from build123d import *

# Parameters (mm, degrees)
SKETCH1_R                                            = 165
SKETCH1_R_2                                          = 132
BOSS_EXTRUDE1_DEPTH                                  = 15
M8_CLEARANCE_HOLE1_D                                 = 9
CIRPATTERN1_COUNT                                    = 6
SKETCH4_R                                            = 10
CUT_EXTRUDE1_DEPTH                                   = 4
CSK_FOR_M10_HEX_SOCKET_COUNTERSUNK_CAP_S_D           = 11
CSK_FOR_M10_HEX_SOCKET_COUNTERSUNK_CAP_S_CSINK_D     = 24.4
CSK_FOR_M10_HEX_SOCKET_COUNTERSUNK_CAP_S_CSINK_ANGLE = 90
CIRPATTERN2_COUNT                                    = 3


with BuildPart() as part:
    # Sketch1 → Boss-Extrude1 (new body)
    with BuildSketch(Plane(origin=(0, 0, 0), x_dir=(1, 0, 0), z_dir=(0, 1, 0))):
        Circle(SKETCH1_R)
        Circle(SKETCH1_R_2, mode=Mode.SUBTRACT)
    extrude(amount=BOSS_EXTRUDE1_DEPTH)

    # M8 Clearance Hole1 (through all)
    with Locations(Plane(origin=(0, 0, 0), x_dir=(-1, 0, 0), z_dir=(0, -1, 0))):
        with Locations((0, 148.5)):
            m8_clearance_hole1 = Hole(M8_CLEARANCE_HOLE1_D / 2)

    # CirPattern1: M8 Clearance Hole1 ×6 about axis
    cirpattern1_axis = Axis((0, 0, 0), (0, 1, 0))
    for i in range(1, CIRPATTERN1_COUNT):
        add(m8_clearance_hole1.rotate(cirpattern1_axis, i * 360 / CIRPATTERN1_COUNT), mode=Mode.SUBTRACT)

    # Sketch4 → Cut-Extrude1 (cut)
    with BuildSketch(Plane.XZ):
        with Locations((-74.25, 128.604772462)):
            Circle(SKETCH4_R)
    cut_extrude1 = extrude(amount=-CUT_EXTRUDE1_DEPTH, mode=Mode.SUBTRACT)

    # CSK for M10 Hex Socket Countersunk Cap Screw1 (through all)
    with Locations(Plane(origin=(0, 15, 0), x_dir=(1, 0, 0), z_dir=(0, 1, 0))):
        with Locations((-74.25, -128.604772462)):
            csk_for_m10_hex_socket_countersunk_cap_s = CounterSinkHole(CSK_FOR_M10_HEX_SOCKET_COUNTERSUNK_CAP_S_D / 2, CSK_FOR_M10_HEX_SOCKET_COUNTERSUNK_CAP_S_CSINK_D / 2, counter_sink_angle=CSK_FOR_M10_HEX_SOCKET_COUNTERSUNK_CAP_S_CSINK_ANGLE)

    # CirPattern2: Cut-Extrude1, CSK for M10 Hex Socket Countersunk Cap Screw1 ×3 about axis
    cirpattern2_axis = Axis((0, 0, 0), (0, 1, 0))
    for i in range(1, CIRPATTERN2_COUNT):
        add(cut_extrude1.rotate(cirpattern2_axis, i * 360 / CIRPATTERN2_COUNT), mode=Mode.SUBTRACT)
        add(csk_for_m10_hex_socket_countersunk_cap_s.rotate(cirpattern2_axis, i * 360 / CIRPATTERN2_COUNT), mode=Mode.SUBTRACT)


solid = part.part
Geometry: final body of the model. Coordinates: model frame, mm. A direction names the side the tool comes from. Give positions to 0.01 mm unless a question says otherwise; leave off trailing zeros. Write each loop counter-clockwise with the first axis right and the second up, starting at its lowest first coordinate (ties: lowest second). Pieces come first, ordered by that corner, then holes.
(1) Mould query, pull axis X, two halves, no side actions, for faces 1 (the flat face through (-123, 15, -50)), 2 (the cylindrical face through (-81.62, 1.972, 135.363)). Classes: released by +X, released by -X, zero draft, split by the parting line, or undercut.
(2) Cut plane D-D, the plane z = 74.25. Return loops of the section in (x, y).
(3) Cut plane B-B, the plane z = 0. Return loops of the section in (x, y).
(4) Cut plane C-C, the plane z = 148.5. Return loops of the section in (x, y), then the cut area to 3 significant figures.
(5) Access query for faces 3 (the flat face through (-70, 4, 124)), 4 (the cylindrical face through (-132.176, 7.605, 76.988)). Directions: +Z, -Z, +X, -X, +Y, -Y. A direction counts if a zero-diameter tool reaches every point of the face in a straight line with its end or side. Return the directions, or none.
(6) First-contact query: P1, Ø4, axis at y = 9, z = 33.5, coming from the -X side; P2, Ø7, axis at x = 0, z = 148.5, coming from the +Y side; P3, Ø5, axis at x = -4.5, y = 12.5, coming from the -Z side; P4, Ø14.5, axis at x = -74.25, z = 128.6, coming from the -Y side. Flat tips, straight axial feed; report the tip coordinate or a pass-through.
(7) Cut plane A-A, the plane x = 0. Return loops of the section in (y, z).
(8) Ray query, line 1 (Z direction, x = 0, y = 9.25); line 2 (X direction, y = 3.25, z = 0); line 3 (Z direction, x = 4, y = 12.5). Return the intervals inside material, ascending.
Values follow:
1. face 1: zero draft
1. face 2: undercut
2. outline: (-147.35, 0) - (-133.1, 0) - (-133.1, 15) - (-147.35, 15) - close; (-124.1, 0) - (-109.14, 0) - (-109.14, 15) - (-124.1, 15) - close; (109.14, 0) - (124.1, 0) - (124.1, 15) - (109.14, 15) - close; (133.1, 0) - (147.35, 0) - (147.35, 15) - (133.1, 15) - close
3. outline: (-165, 0) - (-132, 0) - (-132, 15) - (-165, 15) - close; (132, 0) - (138.5, 0) - (138.5, 4) - (143, 4) - (143, 8.3) - (136.3, 15) - (132, 15) - close; (154, 4) - (158.5, 4) - (158.5, 0) - (165, 0) - (165, 15) - (160.7, 15) - (154, 8.3) - close
4. outline: (-71.92, 0) - (-4.5, 0) - (-4.5, 15) - (-71.92, 15) - close; (4.5, 0) - (71.92, 0) - (71.92, 15) - (4.5, 15) - close
4. area: 2,020 mm2
5. face 3: -Y
5. face 4: +Y, -Y
6. P1: stops at x = -161.97
6. P2: passes through
6. P3: stops at z = -164.99
6. P4: stops at y = 4
7. outline: (0, -165) - (15, -165) - (15, -153) - (0, -153) - close; (0, -144) - (15, -144) - (15, -132) - (0, -132) - close; (0, 132) - (15, 132) - (15, 144) - (0, 144) - close; (0, 153) - (15, 153) - (15, 165) - (0, 165) - close
8. line 1: z = -165 to -153, -144 to -132, 132 to 144, 153 to 165
8. line 2: x = -165 to -132, 132 to 138.5, 158.5 to 165
8. line 3: z = -164.95 to -150.56, -146.44 to -131.94, 131.94 to 146.44, 150.56 to 164.95
